Verification items for the finished model (mm, model axes). Round coordinates to 2 decimals unless told otherwise and drop trailing zeros. Loops run counter-clockwise (first coordinate to the right, second up) from the corner with the lowest first, then second, coordinate; pieces in that order, holes last.
from build123d import *

# Parameters (mm, degrees)
BOSS_EXTRUDE1_DEPTH = 6.25
FILLET1_R           = 10


with BuildPart() as part:
    # Sketch2 → Boss-Extrude1 (new body, symmetric)
    with BuildSketch(Plane(origin=(0, 0, 0), x_dir=(1, 0, 0), z_dir=(0, 1, 0))):
        with BuildLine():
            Line((-515, 150), (-515, -150))
            ThreePointArc((-515, -150), (-340, -240), (-165, -150))
            ThreePointArc((-165, -150), (0, -205), (165, -150))
            Line((165, -150), (165, 150))
            Line((165, 150), (165, 280))
            ThreePointArc((165, 280), (0, 445), (-165, 280))
            Line((-165, 280), (-165, 150))
            ThreePointArc((-165, 150), (-340, 287.869251134), (-515, 150))
        make_face()
    extrude(amount=BOSS_EXTRUDE1_DEPTH, both=True)

    # Fillet1
    fillet1_edges = [part.edges().sort_by_distance(p)[0] for p in [
        (-165, 0, 150),
        (-165, 0, -150),
        (165, 0, 150),
    ]]
    fillet(fillet1_edges, radius=FILLET1_R)


solid = part.part
1. Section check C-C (z = -383). Enter the section's corners in (x, y).
2. Section check A-A (z = -222). Enter the section's corners in (x, y).
3. Gauge pin test, flat ends, axial feed: P1, Ø3, axis at y = -0.5, z = 157, coming from the +X side; P2, Ø1.5, axis at y = -2.5, z = -300.5, coming from the -X side; P3, Ø1, axis at x = -129, y = -1, coming from the +Z side. Record the tip position at first contact, or that the pin passes through.
4. Section check B-B (x = 0). Enter the section's corners in (y, z), then the cut area to 4 significant figures.
5. Release check for a two-part mould opening along X. For faces 1 (the face through (-180, -6.25, -107)), 2 (the face through (0, 0, 205)), 3 (the face through (-347.596, 0.088, 239.866)) record: released by +X, released by -X, zero draft, split by the parting line, or undercut.
6. Scan lines: L1, parallel to Z at x = -5, y = 1; L2, parallel to X at y = 2, z = -205; L3, parallel to Z at x = -341, y = 4.75. Record each from-to range of solid material in increasing order.
Taken from the geometry:
1. outline: (-128.9, -6.25) - (128.9, -6.25) - (128.9, 6.25) - (-128.9, 6.25) - close
2. outline: (-479.19, -6.25) - (-200.81, -6.25) - (-200.81, 6.25) - (-479.19, 6.25) - close; (-165, -6.25) - (165, -6.25) - (165, 6.25) - (-165, 6.25) - close
3. P1: stops at x = 157.4
3. P2: stops at x = -163.81
3. P3: stops at z = 173.13
4. outline: (-6.25, -445) - (6.25, -445) - (6.25, 205) - (-6.25, 205) - close
4. area: 8,125 mm2
5. face 1: zero draft
5. face 2: undercut
5. face 3: undercut
6. L1: z = -444.92 to 204.95
6. L2: x = -491.54 to -188.46, -165 to 165
6. L3: z = -287.87 to 240
